```python
from build123d import *

# Parameters (mm, degrees)
F0_R     = 10
F0_R_2   = 9.5
F0_R_3   = 1
F1_DEPTH = 4
F2_DEPTH = 6
F3_R     = 10
F3_R_2   = 9.5
F3_R_3   = 1
F4_DEPTH = 4
F5_DEPTH = 14
F6_DEPTH = 20


with BuildPart() as f1:
    # F0 (on Front) → F1 (new body)
    with BuildSketch(Plane.XZ):
        Circle(F0_R)
        Circle(F0_R_2, mode=Mode.SUBTRACT)
        Circle(F0_R_2)
        with BuildLine():
            ThreePointArc((3.897114317, 2.25), (4.3466662183, 1.164685703), (4.5, 0))
            ThreePointArc((4.5, 0), (4.3466662183, -1.164685703), (3.897114317, -2.25))
            ThreePointArc((3.897114317, -2.25), (2.25, -3.897114317), (0, -4.5))
            ThreePointArc((0, -4.5), (-2.25, -3.897114317), (-3.897114317, -2.25))
            ThreePointArc((-3.897114317, -2.25), (-4.5, 0), (-3.897114317, 2.25))
            ThreePointArc((-3.897114317, 2.25), (-2.25, 3.897114317), (0, 4.5))
            ThreePointArc((0, 4.5), (2.25, 3.897114317), (3.897114317, 2.25))
        make_face(mode=Mode.SUBTRACT)
        with BuildLine():
            Line((0, 4.5), (3.897114317, 2.25))
            ThreePointArc((3.897114317, 2.25), (2.25, 3.897114317), (0, 4.5))
        make_face()
        with BuildLine():
            Line((-3.897114317, 2.25), (0, 4.5))
            ThreePointArc((0, 4.5), (-2.25, 3.897114317), (-3.897114317, 2.25))
        make_face()
        with BuildLine():
            Line((-3.897114317, -2.25), (-3.897114317, 2.25))
            ThreePointArc((-3.897114317, 2.25), (-4.5, 0), (-3.897114317, -2.25))
        make_face()
        with BuildLine():
            ThreePointArc((-3.897114317, -2.25), (-2.25, -3.897114317), (0, -4.5))
            Line((0, -4.5), (-3.897114317, -2.25))
        make_face()
        with BuildLine():
            ThreePointArc((0, -4.5), (2.25, -3.897114317), (3.897114317, -2.25))
            Line((3.897114317, -2.25), (0, -4.5))
        make_face()
        Polygon((3.897114317, -2.25), (3.897114317, 2.25), (0, 4.5), (-3.897114317, 2.25), (-3.897114317, -2.25), (0, -4.5), align=None)
        Circle(F0_R_3, mode=Mode.SUBTRACT)
        with BuildLine():
            ThreePointArc((3.897114317, -2.25), (4.3466662183, -1.164685703), (4.5, 0))
            ThreePointArc((4.5, 0), (4.3466662183, 1.164685703), (3.897114317, 2.25))
            Line((3.897114317, 2.25), (3.897114317, -2.25))
        make_face()
    extrude(amount=F1_DEPTH)

    # F0 (on Front) → F2 (join)
    with BuildSketch(Plane.XZ):
        Circle(F0_R_2)
        with BuildLine():
            ThreePointArc((3.897114317, 2.25), (4.3466662183, 1.164685703), (4.5, 0))
            ThreePointArc((4.5, 0), (4.3466662183, -1.164685703), (3.897114317, -2.25))
            ThreePointArc((3.897114317, -2.25), (2.25, -3.897114317), (0, -4.5))
            ThreePointArc((0, -4.5), (-2.25, -3.897114317), (-3.897114317, -2.25))
            ThreePointArc((-3.897114317, -2.25), (-4.5, 0), (-3.897114317, 2.25))
            ThreePointArc((-3.897114317, 2.25), (-2.25, 3.897114317), (0, 4.5))
            ThreePointArc((0, 4.5), (2.25, 3.897114317), (3.897114317, 2.25))
        make_face(mode=Mode.SUBTRACT)
        Polygon((3.897114317, -2.25), (3.897114317, 2.25), (0, 4.5), (-3.897114317, 2.25), (-3.897114317, -2.25), (0, -4.5), align=None)
        Circle(F0_R_3, mode=Mode.SUBTRACT)
        with BuildLine():
            Line((-3.897114317, 2.25), (0, 4.5))
            ThreePointArc((0, 4.5), (-2.25, 3.897114317), (-3.897114317, 2.25))
        make_face()
        with BuildLine():
            Line((0, 4.5), (3.897114317, 2.25))
            ThreePointArc((3.897114317, 2.25), (2.25, 3.897114317), (0, 4.5))
        make_face()
        with BuildLine():
            ThreePointArc((3.897114317, -2.25), (4.3466662183, -1.164685703), (4.5, 0))
            ThreePointArc((4.5, 0), (4.3466662183, 1.164685703), (3.897114317, 2.25))
            Line((3.897114317, 2.25), (3.897114317, -2.25))
        make_face()
        with BuildLine():
            Line((-3.897114317, -2.25), (-3.897114317, 2.25))
            ThreePointArc((-3.897114317, 2.25), (-4.5, 0), (-3.897114317, -2.25))
        make_face()
        with BuildLine():
            ThreePointArc((-3.897114317, -2.25), (-2.25, -3.897114317), (0, -4.5))
            Line((0, -4.5), (-3.897114317, -2.25))
        make_face()
        with BuildLine():
            ThreePointArc((0, -4.5), (2.25, -3.897114317), (3.897114317, -2.25))
            Line((3.897114317, -2.25), (0, -4.5))
        make_face()
    extrude(amount=F2_DEPTH)



with BuildPart() as f4:
    # F3 (on face) → F4 (new body)
    with BuildSketch(Plane.XZ.offset(6)):
        Circle(F3_R)
        Circle(F3_R_2, mode=Mode.SUBTRACT)
        Circle(F3_R_2)
        with BuildLine():
            ThreePointArc((3.897114317, 2.25), (4.3466662183, 1.164685703), (4.5, 0))
            ThreePointArc((4.5, 0), (4.3466662183, -1.164685703), (3.897114317, -2.25))
            ThreePointArc((3.897114317, -2.25), (2.25, -3.897114317), (0, -4.5))
            ThreePointArc((0, -4.5), (-2.25, -3.897114317), (-3.897114317, -2.25))
            ThreePointArc((-3.897114317, -2.25), (-4.5, 0), (-3.897114317, 2.25))
            ThreePointArc((-3.897114317, 2.25), (-2.25, 3.897114317), (0, 4.5))
            ThreePointArc((0, 4.5), (2.25, 3.897114317), (3.897114317, 2.25))
        make_face(mode=Mode.SUBTRACT)
        with BuildLine():
            Line((-3.897114317, 2.25), (0, 4.5))
            ThreePointArc((0, 4.5), (-2.25, 3.897114317), (-3.897114317, 2.25))
        make_face()
        with BuildLine():
            Line((-3.897114317, -2.25), (-3.897114317, 2.25))
            ThreePointArc((-3.897114317, 2.25), (-4.5, 0), (-3.897114317, -2.25))
        make_face()
        with BuildLine():
            Line((0, 4.5), (3.897114317, 2.25))
            ThreePointArc((3.897114317, 2.25), (2.25, 3.897114317), (0, 4.5))
        make_face()
        Polygon((3.897114317, -2.25), (3.897114317, 2.25), (0, 4.5), (-3.897114317, 2.25), (-3.897114317, -2.25), (0, -4.5), align=None)
        Circle(F3_R_3, mode=Mode.SUBTRACT)
        with BuildLine():
            ThreePointArc((3.897114317, -2.25), (4.3466662183, -1.164685703), (4.5, 0))
            ThreePointArc((4.5, 0), (4.3466662183, 1.164685703), (3.897114317, 2.25))
            Line((3.897114317, 2.25), (3.897114317, -2.25))
        make_face()
        with BuildLine():
            ThreePointArc((0, -4.5), (2.25, -3.897114317), (3.897114317, -2.25))
            Line((3.897114317, -2.25), (0, -4.5))
        make_face()
        with BuildLine():
            ThreePointArc((-3.897114317, -2.25), (-2.25, -3.897114317), (0, -4.5))
            Line((0, -4.5), (-3.897114317, -2.25))
        make_face()
    extrude(amount=F4_DEPTH)


with BuildPart() as f1_1:
    add(f1.part)

    add(f4.part)  # F5 merges F4
    # F3 (on face) → F5 (join)
    with BuildSketch(Plane.XZ.offset(6)):
        Polygon((3.897114317, -2.25), (3.897114317, 2.25), (0, 4.5), (-3.897114317, 2.25), (-3.897114317, -2.25), (0, -4.5), align=None)
        Circle(F3_R_3, mode=Mode.SUBTRACT)
    extrude(amount=F5_DEPTH)

    # F3 (on face) → F6 (cut)
    with BuildSketch(Plane.XZ.offset(6)):
        Circle(F3_R_3)
    extrude(amount=F6_DEPTH, mode=Mode.SUBTRACT)


solid = f1_1.part
```
The model under review builds one solid part; all positions refer to its coordinate system, in mm. A direction names the side the tool comes from. Round coordinates to 2 decimals unless told otherwise and drop trailing zeros. Loops run counter-clockwise (first coordinate to the right, second up) from the corner with the lowest first, then second, coordinate; pieces in that order, holes last. Notation, with made-up numbers: (78, 79) -> (109, 79) arc R30 cw to (109, 109) -> close; hole circle Ø5 at (47.5, 36). An arc over 180 degrees is marked (long way). Answer as a JSON object with one key per item and string values. Group by question number.
1) For pin 1 Ø12 at (y, z) = (-15.5, 4) entering from +X; pin 2 Ø3.5 at (y, z) = (-16.5, -1) entering from +X; pin 3 Ø1.3 at (y, z) = (-14, -0.5) entering from -X, all flat-tipped, find the tip position at first contact; note any pin that passes through.
2) We need section A-A on z = 0. Write out the cut boundary in (x, y).
3) We need section C-C on z = 3.75. Write out the cut boundary in (x, y), then the cut area to 3 significant figures.
4) For faces 1 (the face through (4.38, -4.99, -8.43)), 2 (the face through (-1.976, -14.93, -3.359)), 3 (the face through (-3.897, -15, 0)), 4 (the face through (1.976, -14.93, 3.359)), list the 3-axis set-ups (+Z, -Z, +X, -X, +Y, -Y) from which the entire face can be reached by the end or side of a thin tool; tool diameter is ignored.
5) We need section D-D on x = -5.75. Write out the cut boundary in (y, z), then the cut area to 3 significant figures.
6) For line 1 (Z direction, x = 0, y = -4.25); line 2 (Z direction, x = 0, y = -8.5); line 3 (Y direction, x = 2.75, z = -4.25), list the stretches that pass through material, from the lowest coordinate up. Write a range as [from, to].
7) Mouldability with a two-part tool opening along X and no side actions: class faces 5 (the face through (1.92, -14.93, -3.39)), 6 (the face through (0, -10, -1)), 7 (the face through (4.3, -10, 0.1)) as released by +X, released by -X, zero draft, split by the parting line, or undercut.
8) We need section B-B on y = -16.5. Write out the cut boundary in (x, z), then the cut area to 3 significant figures.
Result set:
{
 "1": {"pin 1": "x = 9.87", "pin 2": "x = 3.9", "pin 3": "x = -3.9"},
 "2": {"outline": "(-10, -10) -> (-3.9, -10) -> (-3.9, -20) -> (-1, -20) -> (-1, 0) -> (-10, 0) -> (-10, -4) -> (-9.5, -4) -> (-9.5, -6) -> (-10, -6) -> close; (1, -20) -> (3.9, -20) -> (3.9, -10) -> (10, -10) -> (10, -6) -> (9.5, -6) -> (9.5, -4) -> (10, -4) -> (10, 0) -> (1, 0) -> close"},
 "3": {"outline": "(-9.27, -10) -> (-1.3, -10) -> (-1.3, -20) -> (1.3, -20) -> (1.3, -10) -> (9.27, -10) -> (9.27, -6) -> (8.73, -6) -> (8.73, -4) -> (9.27, -4) -> (9.27, 0) -> (-9.27, 0) -> (-9.27, -4) -> (-8.73, -4) -> (-8.73, -6) -> (-9.27, -6) -> close", "area": "209 mm²"},
 "4": {"face 1": "none", "face 2": "-Z, -X, -Y", "face 3": "+Z, -Z, -X, -Y", "face 4": "+Z, +X, -Y"},
 "5": {"outline": "(-10, -8.18) -> (-6, -8.18) -> (-6, -7.56) -> (-4, -7.56) -> (-4, -8.18) -> (0, -8.18) -> (0, 8.18) -> (-4, 8.18) -> (-4, 7.56) -> (-6, 7.56) -> (-6, 8.18) -> (-10, 8.18) -> close", "area": "161 mm²"},
 "6": {"line 1": "[-9.5, -1], [1, 9.5]", "line 2": "[-10, -1], [1, 10]", "line 3": "[-10, 0]"},
 "7": {"face 5": "released by +X", "face 6": "undercut", "face 7": "zero draft"},
 "8": {"outline": "(-3.9, -2.25) -> (0, -4.5) -> (3.9, -2.25) -> (3.9, 2.25) -> (0, 4.5) -> (-3.9, 2.25) -> close; hole circle Ø2 at (0, 0)", "area": "49.5 mm²"}
}
